```python
from build123d import *

# Parameters (mm, degrees)
PAD_DEPTH       = 8
SKETCH001_R     = 11
POCKET_DEPTH    = 6
SKETCH002_R     = 5
POCKET001_DEPTH = 2
SKETCH003_W     = 30
SKETCH003_H     = 6
PAD001_DEPTH    = 15
SKETCH004_R     = 2.3
POCKET002_DEPTH = 6


with BuildPart() as part:
    # Sketch → Pad (new body)
    with BuildSketch(Plane.XY):
        with BuildLine():
            ThreePointArc((15, 20.679889), (0, 35.679889), (-15, 20.679889))
            Line((-15, 20.679889), (-15, 0.179889))
            Line((-15, 0.179889), (15, 0.179889))
            Line((15, 20.679889), (15, 0.179889))
        make_face()
    extrude(amount=PAD_DEPTH)

    # Sketch001 (on Face6 of Pad) → Pocket (cut)
    with BuildSketch(Plane.XY.offset(8)):
        with Locations((0, 20.679889)):
            Circle(SKETCH001_R)
    extrude(amount=-POCKET_DEPTH, mode=Mode.SUBTRACT)

    # Sketch002 (on Face4 of Pocket) → Pocket001 (cut)
    with BuildSketch(Plane(origin=(0, 0, 0), x_dir=(1, 0, 0), z_dir=(0, 0, -1))):
        with Locations((0, -20.679889)):
            Circle(SKETCH002_R)
    extrude(amount=-POCKET001_DEPTH, mode=Mode.SUBTRACT)

    # Sketch003 (on Face5 of Pocket001) → Pad001 (join)
    with BuildSketch(Plane.XY.offset(8)):
        with Locations((0, 3.179889)):
            Rectangle(SKETCH003_W, SKETCH003_H)
    extrude(amount=PAD001_DEPTH)

    # Sketch004 (on Face12 of Pad001) → Pocket002 (cut)
    with BuildSketch(Plane.XZ.offset(-0.179889)):
        with Locations((-10.2, 12.8)):
            Circle(SKETCH004_R)
        with Locations((10.2, 12.8)):
            Circle(SKETCH004_R)
    extrude(amount=-POCKET002_DEPTH, mode=Mode.SUBTRACT)


solid = part.part
```
Check sheet for the modelled part. Datum: model origin and axes. Units: mm. A direction names the side the tool comes from. Coordinates: 2 decimals unless noted, no trailing zeros. Loops run counter-clockwise (first coordinate to the right, second up) from the corner with the lowest first, then second, coordinate; pieces in that order, holes last.
1) Sectioned sample at D-D (y = 18.5). Record the boundary of the cut face in (x, z), and give its area (3 significant figures).
2) Release check for a two-part mould opening along X. For faces 4 (the face through (0.33, 35.676, 3.944)), 5 (the face through (0, 6.18, 15)), 6 (the face through (2.3, 15.9, 2)) record: released by +X, released by -X, zero draft, split by the parting line, or undercut.
3) Access from +Z, -Z, +X, -X, +Y, -Y to the whole of each face (thin tool, end or side, straight path). Record for faces 1 (the face through (0, 14, 0)), 2 (the face through (6, 11, 8)), 3 (the face through (-2.38, 9.94, 5.04)).
4) Sectioned sample at A-A (z = 12.8). Record the boundary of the cut face in (x, y).
5) Sectioned sample at C-C (x = 0). Record the boundary of the cut face in (y, z).
6) Sectioned sample at B-B (y = 4.5). Record the boundary of the cut face in (x, z).
7) Gauge pin test, flat ends, axial feed: pin 1 (4 mm diameter, centred on x = 10.2, z = 12.8, fed in from -Y); pin 2 (6 mm diameter, centred on x = -7.5, z = 3.5, fed in from +Y); pin 3 (6 mm diameter, centred on x = -10.2, z = 12.8, fed in from +Y); pin 4 (1.5 mm diameter, centred on x = 9, y = 10, fed in from +Z). Record the tip position at first contact, or that the pin passes through.
8) Material ranges on probe 1 along Y at (x, z) = (0, 4.3); probe 2 along Y at (x, z) = (0, 1.05); probe 3 along Y at (x, z) = (10.25, 16.25), recorded low to high.
Check sheet entries:
1. outline: (-15, 0) - (-4.5, 0) - (-4.5, 2) - (-10.78, 2) - (-10.78, 8) - (-15, 8) - close; (4.5, 0) - (15, 0) - (15, 8) - (10.78, 8) - (10.78, 2) - (4.5, 2) - close
1. area: 92.6 mm2
2. face 4: split by the parting line
2. face 5: zero draft
2. face 6: undercut
3. face 1: -Z, +X, -X, +Y, -Y
3. face 2: +Z, +X, -X, +Y
3. face 3: +Z
4. outline: (-15, 0.18) - (-12.5, 0.18) - (-12.5, 6.18) - (-15, 6.18) - close; (-7.9, 0.18) - (7.9, 0.18) - (7.9, 6.18) - (-7.9, 6.18) - close; (12.5, 0.18) - (15, 0.18) - (15, 6.18) - (12.5, 6.18) - close
5. outline: (0.18, 0) - (15.68, 0) - (15.68, 2) - (9.68, 2) - (9.68, 8) - (6.18, 8) - (6.18, 23) - (0.18, 23) - close; (25.68, 0) - (35.68, 0) - (35.68, 8) - (31.68, 8) - (31.68, 2) - (25.68, 2) - close
6. outline: (-15, 0) - (15, 0) - (15, 23) - (-15, 23) - close; hole circle Ø4.6 at (-10.2, 12.8); hole circle Ø4.6 at (10.2, 12.8)
7. pin 1: passes through
7. pin 2: stops at y = 34.99
7. pin 3: stops at y = 6.18
7. pin 4: stops at z = 8
8. probe 1: y = 0.18 to 9.68, 31.68 to 35.68
8. probe 2: y = 0.18 to 15.68, 25.68 to 35.68
8. probe 3: y = 0.18 to 6.18
